```python
from build123d import *

# Parameters (mm, degrees)
F0_W      = 385
F0_H      = 315
F1_DEPTH  = 345
F2_W      = 60
F2_H      = 75
F3_DEPTH  = 10
F4_R      = 10
F5_W      = 28
F5_H      = 28
F6_DEPTH  = 4
F7_R      = 10.65
F8_DEPTH  = 40
F9_R      = 10.65
F10_DEPTH = 40


with BuildPart() as f1:
    # F0 (on Front) → F1 (new body)
    with BuildSketch(Plane.XZ):
        with Locations((192.5, 157.5)):
            Rectangle(F0_W, F0_H)
    extrude(amount=F1_DEPTH)

    # F2 (on face) → F3 (join)
    with BuildSketch(Plane.XZ.offset(345)):
        with Locations((337, 55.5)):
            Rectangle(F2_W, F2_H)
    extrude(amount=F3_DEPTH)

    # F4
    f4_edges = [f1.edges().sort_by_distance(p)[0] for p in [
        (367, -350, 93),
        (367, -350, 18),
        (307, -350, 93),
        (307, -350, 18),
    ]]
    fillet(f4_edges, radius=F4_R)

    # F5 (on face) → F6 (cut)
    with BuildSketch(Plane.XZ.offset(355)):
        with Locations((338, 55)):
            Rectangle(F5_W, F5_H)
    extrude(amount=-F6_DEPTH, mode=Mode.SUBTRACT)

    # F7 (on face) → F8 (join)
    with BuildSketch(Plane(origin=(0, 0, 0), x_dir=(1, 0, 0), z_dir=(0, 0, -1))):
        with Locations((98.254092, 102.251634)):
            Circle(F7_R)
    extrude(amount=F8_DEPTH)

    # F9 (on face) → F10 (join)
    with BuildSketch(Plane(origin=(0, 0, 0), x_dir=(1, 0, 0), z_dir=(0, 0, -1))):
        with Locations((273.860931, 81.706926)):
            Circle(F9_R)
    extrude(amount=F10_DEPTH)


solid = f1.part
```
Geometry: final body of the model. Coordinates: model frame, mm. A direction names the side the tool comes from. Coordinates: 2 decimals unless noted, no trailing zeros. Loops run counter-clockwise (first coordinate to the right, second up) from the corner with the lowest first, then second, coordinate; pieces in that order, holes last. Notation, with made-up numbers: (-36, 40.25) -> (22, 40.25) arc R31 cw to (22, 76.25) -> close; hole circle Ø10 at (78, -39.5). An arc over 180 degrees is marked (long way). Use a Markdown table: item, result. Add a question column.
(1) Pin query (flat end, axial travel): pin 1 Ø3 at (x, y) = (333.5, -354) entering from -Z; pin 2 Ø5 at (y, z) = (-349.5, 68.5) entering from -X; pin 3 Ø4 at (x, y) = (279, -301.5) entering from -Z. Return the tip coordinate at first contact, or that it passes through.
(2) Access query for faces 1 (the cylindrical face through (364.15, -350.07, 89.99)), 2 (the cylindrical face through (363.99, -350.07, 20.85)), 3 (the cylindrical face through (263.22, -82.18, -19.72)). Directions: +Z, -Z, +X, -X, +Y, -Y. A direction counts if a zero-diameter tool reaches every point of the face in a straight line with its end or side. Return the directions, or none.
(3) Section query C-C, the plane z = -8. Return loops of the section in (x, y), plus the area to 3 significant figures.
(4) Section query A-A, the plane z = 203. Return loops of the section in (x, y), plus the area to 3 significant figures.
(5) Line query: line 1 along Z through (x, y) = (142.5, -251); line 2 along Y through (x, z) = (82, 13). Output: solid intervals per line, ascending.
(6) Section query B-B, the plane x = 148.5. Return loops of the section in (y, z).
Answer:
| question | item | result |
|---|---|---|
| 1 | pin 1 | stops at z = 18 |
| 1 | pin 2 | stops at x = 307 |
| 1 | pin 3 | stops at z = 0 |
| 2 | face 1 | +Z, +X, -Y |
| 2 | face 2 | -Z, +X, -Y |
| 2 | face 3 | -Z |
| 3 | outline | circle Ø21.3 at (98.25, -102.25); circle Ø21.3 at (273.86, -81.71) |
| 3 | area | 713 mm^2 |
| 4 | outline | (0, -345) -> (385, -345) -> (385, 0) -> (0, 0) -> close |
| 4 | area | 133,000 mm^2 |
| 5 | line 1 | z = 0 to 315 |
| 5 | line 2 | y = -345 to 0 |
| 6 | outline | (-345, 0) -> (0, 0) -> (0, 315) -> (-345, 315) -> close |
